CAD build for the part. Positions are in the model's coordinates, mm. A direction names the side the tool comes from. Give positions to 0.01 mm unless a question says otherwise; leave off trailing zeros. Loops run counter-clockwise (first coordinate to the right, second up) from the corner with the lowest first, then second, coordinate; pieces in that order, holes last.
```python
from build123d import *

# Parameters (mm, degrees)
SKETCH_W     = 200
SKETCH_H     = 130
SKETCH_R     = 35
SKETCH_R_2   = 1.5625
PAD_DEPTH    = 10
SKETCH001_R  = 40
POCKET_DEPTH = 7.5
FILLET_R     = 3


with BuildPart() as part:
    # Sketch → Pad (new body)
    with BuildSketch(Plane.XY):
        with Locations((100, 65)):
            Rectangle(SKETCH_W, SKETCH_H)
        with Locations((100, 65)):
            Circle(SKETCH_R, mode=Mode.SUBTRACT)
        with Locations((45, 115)):
            Circle(SKETCH_R_2, mode=Mode.SUBTRACT)
        with Locations((45, 15)):
            Circle(SKETCH_R_2, mode=Mode.SUBTRACT)
        with Locations((155, 115)):
            Circle(SKETCH_R_2, mode=Mode.SUBTRACT)
        with Locations((155, 15)):
            Circle(SKETCH_R_2, mode=Mode.SUBTRACT)
        with Locations((185, 30)):
            Circle(SKETCH_R_2, mode=Mode.SUBTRACT)
        with Locations((135.353085, 100.338453)):
            Circle(SKETCH_R_2, mode=Mode.SUBTRACT)
        with Locations((64.627773, 29.642413)):
            Circle(SKETCH_R_2, mode=Mode.SUBTRACT)
        with Locations((64.64463, 100.35537)):
            Circle(SKETCH_R_2, mode=Mode.SUBTRACT)
        with Locations((135.352442, 29.63292)):
            Circle(SKETCH_R_2, mode=Mode.SUBTRACT)
        with Locations((175, 20)):
            Circle(SKETCH_R_2, mode=Mode.SUBTRACT)
        with Locations((175, 40)):
            Circle(SKETCH_R_2, mode=Mode.SUBTRACT)
        with Locations((185, 50)):
            Circle(SKETCH_R_2, mode=Mode.SUBTRACT)
        with Locations((175, 90)):
            Circle(SKETCH_R_2, mode=Mode.SUBTRACT)
        with Locations((175, 110)):
            Circle(SKETCH_R_2, mode=Mode.SUBTRACT)
        with Locations((185, 80)):
            Circle(SKETCH_R_2, mode=Mode.SUBTRACT)
        with Locations((185, 100)):
            Circle(SKETCH_R_2, mode=Mode.SUBTRACT)
        with Locations((15, 30)):
            Circle(SKETCH_R_2, mode=Mode.SUBTRACT)
        with Locations((25, 20)):
            Circle(SKETCH_R_2, mode=Mode.SUBTRACT)
        with Locations((25, 40)):
            Circle(SKETCH_R_2, mode=Mode.SUBTRACT)
        with Locations((15, 50)):
            Circle(SKETCH_R_2, mode=Mode.SUBTRACT)
        with Locations((25, 90)):
            Circle(SKETCH_R_2, mode=Mode.SUBTRACT)
        with Locations((25, 110)):
            Circle(SKETCH_R_2, mode=Mode.SUBTRACT)
        with Locations((15, 80)):
            Circle(SKETCH_R_2, mode=Mode.SUBTRACT)
        with Locations((15, 100)):
            Circle(SKETCH_R_2, mode=Mode.SUBTRACT)
    extrude(amount=PAD_DEPTH)

    # Sketch001 (on Face31 of Pad) → Pocket (cut)
    with BuildSketch(Plane.XY.offset(10)):
        with Locations((100, 65)):
            Circle(SKETCH001_R)
    extrude(amount=-POCKET_DEPTH, mode=Mode.SUBTRACT)

    # Fillet
    fillet_edges = [part.edges().sort_by_distance(p)[0] for p in [
        (200, 0, 5),
        (200, 130, 5),
        (0, 0, 5),
        (0, 130, 5),
    ]]
    fillet(fillet_edges, radius=FILLET_R)


solid = part.part
```
1. Probe line 1 along Y through (x, z) = (175, 5); line 2 along Y through (x, z) = (185, 7); line 3 along X through (y, z) = (114, 3). List the from-to ranges inside material, lowest first.
Responses:
line 1: y = 0 to 18.44, 21.56 to 38.44, 41.56 to 88.44, 91.56 to 108.44, 111.56 to 130
line 2: y = 0 to 28.44, 31.56 to 48.44, 51.56 to 78.44, 81.56 to 98.44, 101.56 to 130
line 3: x = 0 to 43.8, 46.2 to 153.8, 156.2 to 200
2. Saw through at A-A, the plane x = 93. List the corners of the cut face in (y, z), and give its area (3 significant figures).
Responses:
outline: (0, 0) - (30.71, 0) - (30.71, 2.5) - (25.62, 2.5) - (25.62, 10) - (0, 10) - close; (99.29, 0) - (130, 0) - (130, 10) - (104.38, 10) - (104.38, 2.5) - (99.29, 2.5) - close
area: 538 mm2
3. Tool access for faces 4 (the face through (99.8, 29.6, 2.5)), 5 (the face through (99, 0, 5)): list every direction of +Z, -Z, +X, -X, +Y, -Y with a clear straight run to the whole face (end or side of a thin tool).
Responses:
face 4: +Z
face 5: +Z, -Z, +X, -X, -Y
4. Saw through at C-C, the plane y = 75. List the corners of the cut face in (x, z).
Responses:
outline: (0, 0) - (66.46, 0) - (66.46, 2.5) - (61.27, 2.5) - (61.27, 10) - (0, 10) - close; (133.54, 0) - (200, 0) - (200, 10) - (138.73, 10) - (138.73, 2.5) - (133.54, 2.5) - close
5. Saw through at B-B, the plane z = 4.5. Count the separate pieces of the cut face and the enclosed holes in it, and give its area (3 significant figures).
Responses:
separate pieces: 1
enclosed holes: 25
area: 20,800 mm2
6. Pull direction Y, two halves, no side cores. Call faces 1 (the face through (118.82, 94.51, 1.23)), 2 (the face through (99, 130, 5)), 3 (the face through (76, 95, 0)): released by +Y, released by -Y, zero draft, split by the parting line, or undercut.
Responses:
face 1: undercut
face 2: released by +Y
face 3: zero draft
